```python
from build123d import *

# Parameters (mm, degrees)
BOSS_EXTRUDE1_DEPTH = 5
BOSS_EXTRUDE2_REACH = 322
SKETCH2_W           = 10
SKETCH2_H           = 15
SKETCH3_W           = 9.887044096
SKETCH3_H           = 15
BOSS_EXTRUDE3_DEPTH = 89.560962
SKETCH4_R           = 2.5
CUT_EXTRUDE1_DEPTH  = 320
SKETCH5_W           = 360
SKETCH5_H           = 7.556477952
BOSS_EXTRUDE4_DEPTH = 320
BOSS_EXTRUDE5_DEPTH = 30
CUT_EXTRUDE2_DEPTH  = 30


with BuildPart() as part:
    # Sketch1 → Boss-Extrude1 (new body)
    with BuildSketch(Plane.XY):
        Polygon((175.89978938, 161.770375321), (-184.213166524, 161.770375321), (-184.213166524, -158.229624679), (175.89978938, -158.229624679), (185.786833476, -158.229624679), (185.786833476, -68.668662794), (175.89978938, -68.668662794), (175.89978938, 72.40143746), (185.786833476, 72.209413435), (185.786833476, 161.770375321), align=None)
    extrude(amount=BOSS_EXTRUDE1_DEPTH)

    # Boss-Extrude2: up to this face of the body (flat: up to its plane)
    boss_extrude2_end = Plane(part.part.faces().sort_by_distance((180.843311428, 72.305425448, 2.5))[0])
    # Sketch2 → Boss-Extrude2 (add, up to the picked face)
    with BuildSketch(Plane(origin=(0, 161.770375321, 0), x_dir=(1, 0, 0), z_dir=(0, 1, 0)), mode=Mode.PRIVATE) as boss_extrude2_sk1:
        with Locations((180.786833476, -7.5)):
            Rectangle(SKETCH2_W, SKETCH2_H)
    boss_extrude2_tool1 = split(extrude(boss_extrude2_sk1.sketch, amount=-BOSS_EXTRUDE2_REACH, mode=Mode.PRIVATE), bisect_by=boss_extrude2_end, keep=Keep.BOTH, mode=Mode.PRIVATE)
    add(boss_extrude2_tool1.solids().sort_by_distance((180.786833, 161.770375, 7.5))[0])

    # Sketch3 → Boss-Extrude3 (add)
    with BuildSketch(Plane.XZ.offset(158.229624679)):
        with Locations((180.843311428, 7.5)):
            Rectangle(SKETCH3_W, SKETCH3_H)
    extrude(amount=-BOSS_EXTRUDE3_DEPTH)

    # Sketch4 → Cut-Extrude1 (cut)
    with BuildSketch(Plane(origin=(0, 161.770375321, 0), x_dir=(1, 0, 0), z_dir=(0, 1, 0))):
        with Locations((180.843311428, -7.5)):
            Circle(SKETCH4_R)
        with BuildLine():
            Line((180.843311428, -12.556477952), (174.586681461, -12.556477952))
            Line((174.586681461, -12.556477952), (174.586681461, -18.742126007))
            Line((174.586681461, -18.742126007), (187.888181218, -19.204340284))
            Line((187.888181218, -19.204340284), (188.294895745, -7.5))
            Line((188.294895745, -7.5), (185.89978938, -7.5))
            ThreePointArc((185.89978938, -7.5), (184.418781277, -11.075469849), (180.843311428, -12.556477952))
        make_face()
    extrude(amount=-CUT_EXTRUDE1_DEPTH, mode=Mode.SUBTRACT)

    # Sketch5 → Boss-Extrude4 (add)
    with BuildSketch(Plane(origin=(0, 161.770375321, 0), x_dir=(1, 0, 0), z_dir=(0, 1, 0))):
        with Locations((-4.213166524, -8.778238976)):
            Rectangle(SKETCH5_W, SKETCH5_H)
    extrude(amount=-BOSS_EXTRUDE4_DEPTH)

    # Sketch6 → Boss-Extrude5 (add)
    with BuildSketch(Plane.XY.offset(12.556477952)):
        with BuildLine():
            Line((-127.887955303, 37.634320881), (-127.887955303, -52.365679119))
            ThreePointArc((-127.887955303, -52.365679119), (-137.887955303, -62.365679119), (-147.887955303, -52.365679119))
            Line((-147.887955303, -52.365679119), (-147.887955303, 37.634320881))
            ThreePointArc((-147.887955303, 37.634320881), (-137.887955303, 47.634320881), (-127.887955303, 37.634320881))
        make_face()
    extrude(amount=BOSS_EXTRUDE5_DEPTH)

    # Sketch7 → Cut-Extrude2 (cut)
    with BuildSketch(Plane.ZY.offset(147.887955303)):
        with BuildLine():
            Line((12.556477952, 47.634320881), (30.556477952, 47.634320881))
            ThreePointArc((30.556477952, 47.634320881), (39.041759326, 44.119602255), (42.556477952, 35.634320881))
            Line((42.556477952, 35.634320881), (42.556477952, -50.365679119))
            ThreePointArc((42.556477952, -50.365679119), (39.041759326, -58.850960494), (30.556477952, -62.365679119))
            Line((30.556477952, -62.365679119), (12.556477952, -62.365679119))
            Line((12.556477952, -62.365679119), (12.556477952, -84.546006254))
            Line((12.556477952, -84.546006254), (75.194935331, -84.546006254))
            Line((75.194935331, -84.546006254), (75.194935331, -40.351574991))
            Line((75.194935331, -40.351574991), (70.864672609, 64.078414926))
            Line((70.864672609, 64.078414926), (12.556477952, 64.078414926))
            Line((12.556477952, 64.078414926), (12.556477952, 47.634320881))
        make_face()
        with BuildLine():
            Line((32.556477952, -7.365679119), (32.556477952, 27.634320881))
            ThreePointArc((32.556477952, 27.634320881), (29.627545764, 34.705388692), (22.556477952, 37.634320881))
            Line((22.556477952, 37.634320881), (12.556477952, 37.634320881))
            Line((12.556477952, 37.634320881), (12.556477952, -52.365679119))
            Line((12.556477952, -52.365679119), (22.556477952, -52.365679119))
            ThreePointArc((22.556477952, -52.365679119), (29.627545764, -49.436746931), (32.556477952, -42.365679119))
            Line((32.556477952, -42.365679119), (32.556477952, -7.365679119))
        make_face()
    extrude(amount=-CUT_EXTRUDE2_DEPTH, mode=Mode.SUBTRACT)


solid = part.part
```
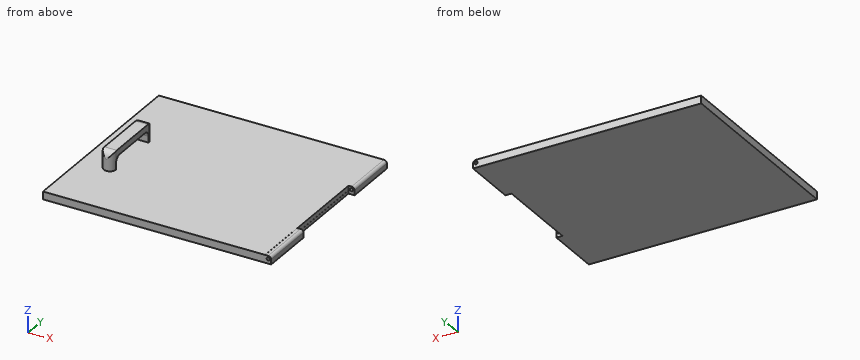
Can you work these out from the model? Positions are in its coordinate system, mm. Coordinates: 2 decimals unless noted, no trailing zeros. Loops run counter-clockwise (first coordinate to the right, second up) from the corner with the lowest first, then second, coordinate; pieces in that order, holes last.
Item 1: Suppose I cut it at D-D (x = 125). Please give me the cut outline in (y, z), then the cut area to 3 significant figures.
Answers below:
outline: (-158.23, 0) - (161.77, 0) - (161.77, 12.56) - (-158.23, 12.56) - close
area: 4,020 mm2
Item 2: I'm going to push flat-ended pins straight in: pin 1 (4 mm diameter, centred on x = 33.5, y = 14.5, fed in from +Z); pin 2 (10 mm diameter, centred on y = -19, z = 28.5, fed in from +X); pin 3 (5 mm diameter, centred on x = -134, z = 19, fed in from -Y). Where does each tip first touch, or does it pass through?
Answers below:
pin 1: stops at z = 12.56
pin 2: stops at x = -127.89
pin 3: stops at y = -62.27
Item 3: Suppose I cut it at B-B (y = 60). Please give me the cut outline in (x, z).
Answers below:
outline: (-184.21, 0) - (175.9, 0) - (175.9, 5) - (175.79, 5) - (175.79, 12.56) - (-184.21, 12.56) - close
Item 4: Please list where these lines run through material, in increasing order: L1, parallel to X at y = 108, z = 7; L2, parallel to X at y = 106, z = 7.5; L3, parallel to Z at x = -163, y = -46.
Answers below:
L1: x = -184.21 to 178.39, 183.29 to 185.79
L2: x = -184.21 to 178.34, 183.34 to 185.79
L3: z = 0 to 12.56
Item 5: Suppose I cut it at A-A (y = 2). Please give me the cut outline in (x, z).
Answers below:
outline: (-184.21, 0) - (175.9, 0) - (175.9, 5) - (175.79, 5) - (175.79, 12.56) - (-184.21, 12.56) - close; (-147.89, 32.56) - (-127.89, 32.56) - (-127.89, 42.56) - (-147.89, 42.56) - close
Item 6: Suppose I cut it at C-C (z = 38). Please give me the cut outline in (x, y).
Answers below:
outline: (-147.89, -52.37) arc R10 ccw to (-144.6, -59.78) - (-131.18, -59.78) arc R10 ccw to (-127.89, -52.37) - (-127.89, 37.63) arc R10 ccw to (-131.18, 45.05) - (-144.6, 45.05) arc R10 ccw to (-147.89, 37.63) - close
